from build123d import *

# Parameters (mm, degrees)
SKETCH011_R          = 11
SKETCH011_R_2        = 3.5
PAD006_DEPTH         = 12.5
POCKET003_DEPTH      = 2.5
SKETCH013_R          = 1.25
POCKET004_DEPTH      = 92.325808
POCKET004_DEPTH_BACK = 92.325808
POLARPATTERN_COUNT   = 15
CHAMFER_SIZE         = 0.5


with BuildPart() as part:
    # Sketch011 → Pad006 (new body, symmetric)
    with BuildSketch(Plane.XY):
        Circle(SKETCH011_R)
        Circle(SKETCH011_R_2, mode=Mode.SUBTRACT)
    extrude(amount=PAD006_DEPTH, both=True)

    # Sketch012 → Pocket003 (cut, symmetric)
    with BuildSketch(Plane.XY):
        Polygon((0, 5.888973), (-5.1, 2.944486), (-5.1, -2.944486), (0, -5.888973), (5.1, -2.944486), (5.1, 2.944486), align=None)
    extrude(amount=POCKET003_DEPTH, both=True, mode=Mode.SUBTRACT)

    # Sketch013 → Pocket004 (cut, two sides)
    with BuildSketch(Plane.XY) as pocket004_sk:
        with Locations((11.5, 0)):
            Circle(SKETCH013_R)
    pocket004 = extrude(amount=-POCKET004_DEPTH, mode=Mode.SUBTRACT) + extrude(pocket004_sk.sketch, amount=POCKET004_DEPTH_BACK, mode=Mode.SUBTRACT)

    # PolarPattern: Pocket004 ×15 about axis
    polarpattern_axis = Axis((0, 0, 0), (0, 0, 1))
    for i in range(1, POLARPATTERN_COUNT):
        add(pocket004.rotate(polarpattern_axis, i * 360 / POLARPATTERN_COUNT), mode=Mode.SUBTRACT)

    # Chamfer
    chamfer_edges = [part.edges().sort_by_distance(p)[0] for p in [
        (10.25, 0, 12.5),
        (10.759624, -2.287029, 12.5),
        (9.363841, -4.169051, 12.5),
        (8.899187, -6.465638, 12.5),
        (6.858589, -7.617234, 12.5),
        (5.5, -9.526279, 12.5),
        (3.167424, -9.748329, 12.5),
        (1.149813, -10.939741, 12.5),
        (-1.071417, -10.193849, 12.5),
        (-3.399187, -10.461622, 12.5),
        (-5.125, -8.87676, 12.5),
        (-7.360437, -8.174593, 12.5),
        (-8.292424, -6.024799, 12.5),
        (-10.049, -4.474103, 12.5),
        (-10.026013, -2.131095, 12.5),
        (-11, 0, 12.5),
        (-10.026013, 2.131095, 12.5),
        (-10.049, 4.474103, 12.5),
        (-8.292424, 6.024799, 12.5),
        (-7.360437, 8.174593, 12.5),
        (-5.125, 8.87676, 12.5),
        (-3.399187, 10.461622, 12.5),
        (-1.071417, 10.193849, 12.5),
        (1.149813, 10.939741, 12.5),
        (3.167424, 9.748329, 12.5),
        (5.5, 9.526279, 12.5),
        (6.858589, 7.617234, 12.5),
        (8.899187, 6.465638, 12.5),
        (9.363841, 4.169051, 12.5),
        (10.759624, 2.287029, 12.5),
        (-3.5, 0, 12.5),
        (10.25, 0, -12.5),
        (10.759624, -2.287029, -12.5),
        (9.363841, -4.169051, -12.5),
        (8.899187, -6.465638, -12.5),
        (6.858589, -7.617234, -12.5),
        (5.5, -9.526279, -12.5),
        (3.167424, -9.748329, -12.5),
        (1.149813, -10.939741, -12.5),
        (-1.071417, -10.193849, -12.5),
        (-3.399187, -10.461622, -12.5),
        (-5.125, -8.87676, -12.5),
        (-7.360437, -8.174593, -12.5),
        (-8.292424, -6.024799, -12.5),
        (-10.049, -4.474103, -12.5),
        (-10.026013, -2.131095, -12.5),
        (-11, 0, -12.5),
        (-10.026013, 2.131095, -12.5),
        (-10.049, 4.474103, -12.5),
        (-8.292424, 6.024799, -12.5),
        (-7.360437, 8.174593, -12.5),
        (-5.125, 8.87676, -12.5),
        (-3.399187, 10.461622, -12.5),
        (-1.071417, 10.193849, -12.5),
        (1.149813, 10.939741, -12.5),
        (3.167424, 9.748329, -12.5),
        (5.5, 9.526279, -12.5),
        (6.858589, 7.617234, -12.5),
        (8.899187, 6.465638, -12.5),
        (9.363841, 4.169051, -12.5),
        (10.759624, 2.287029, -12.5),
        (-3.5, 0, -12.5),
    ]]
    chamfer(chamfer_edges, length=CHAMFER_SIZE)


with BuildPart() as part_1:
    # Body002 placement: moved
    add(part.part.moved(Location((0, 0, -53))))


solid = part_1.part
The listing builds one solid part. Answer for the finished solid, in the listing's coordinates (mm). A direction names the side the tool comes from. Coordinates: 2 decimals unless noted, no trailing zeros. Loops run counter-clockwise (first coordinate to the right, second up) from the corner with the lowest first, then second, coordinate; pieces in that order, holes last. Notation, with made-up numbers: M 15.25,-7.75 L 19.25,-7.75 A17 ccw 19.25,20.25 Z; hole C -39,-16 d3. An arc over 180 degrees is marked long. Answer in a Markdown table with one row per item.
1) Determine the mould class of faces 3 (the cylindrical face through (3.233, -1.341, -60.316)), 4 (the cylindrical face through (9.356, 4.187, -52.832)), 5 (the conical face through (-9.817, 4.389, -40.753)) for opening direction X: released by +X, released by -X, zero draft, split by the parting line, or undercut.
Answers below:
| item | result |
|---|---|
| face 3 | undercut |
| face 4 | released by +X |
| face 5 | released by -X |
2) Given pin 1 (4 mm diameter, centred on x = 6.5, z = -48, fed in from -Y); pin 2 (2.5 mm diameter, centred on y = 0, z = -52, fed in from +X), each flat-ended and moving along its own axis, determine where each tip first touches the part or whether it passes through.
Answers below:
| item | result |
|---|---|
| pin 1 | y = -10.04 |
| pin 2 | x = 10.94 |
3) Which of the six approach directions +Z, -Z, +X, -X, +Y, -Y give full straight-line access (tool end or side, diameter ignored) to faces 1 (the flat face through (-2.586, -4.396, -52.965)), 2 (the conical face through (9.249, -4.094, -65.135))?
Answers below:
| item | result |
|---|---|
| face 1 | none |
| face 2 | -Z, +X |
4) Find the intervals of material crossed by probe 1 along Z at (x, y) = (-3.25, 2.5); probe 2 along Y at (x, z) = (0, -47.75); probe 3 along Y at (x, z) = (7.25, -64.5), in increasing order.
Answers below:
| item | result |
|---|---|
| probe 1 | -65.5 to -55.5, -50.5 to -40.5 |
| probe 2 | -11 to -3.5, 3.5 to 11 |
| probe 3 | -7.38 to 7.38 |
5) Find section A-A (y = 0). Determine the outline of the cut face in (x, z).
Answers below:
| item | result |
|---|---|
| outline | M -11,-65 L -10.5,-65.5 L -4,-65.5 L -3.5,-65 L -3.5,-55.5 L -5.1,-55.5 L -5.1,-50.5 L -3.5,-50.5 L -3.5,-41 L -4,-40.5 L -10.5,-40.5 L -11,-41 Z; M 3.5,-65 L 4,-65.5 L 9.75,-65.5 L 10.25,-65 L 10.25,-41 L 9.75,-40.5 L 4,-40.5 L 3.5,-41 L 3.5,-50.5 L 5.1,-50.5 L 5.1,-55.5 L 3.5,-55.5 Z |
